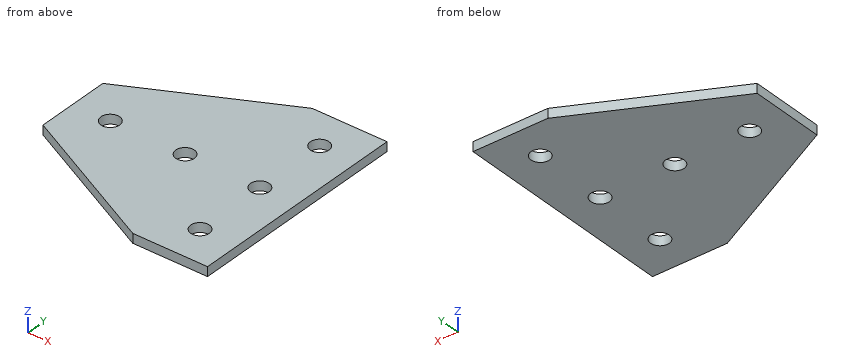
Autodesk Inventor part; units mm, degrees
ref_plane "YZ Plane" through (0, 0, 0) normal (1, 0, 0) x (0, 1, 0)
ref_plane "XZ Plane" through (0, 0, 0) normal (0, 1, 0) x (-1, 0, 0)
ref_plane "XY Plane" through (0, 0, 0) normal (0, 0, 1) x (1, 0, 0)
sketch "Sketch1" plane through (0, 0, 0) normal (0, 0, 1) x (1, 0, 0)
  line L0 (0, 0) -> (0, -76.2)
  line L1 (0, 0) -> (76.2, 0) construction
  line L2 (0, 0) -> (-25.4, 0)
  line L3 (-25.4, 0) -> (-76.2, -25.4)
  line L4 (-76.2, -25.4) -> (-76.2, -50.8)
  line L5 (-76.2, -50.8) -> (-25.4, -76.2)
  line L6 (-25.4, -76.2) -> (0, -76.2)
  circle A0 centre (-12.7, -12.7) radius 3.175
  circle A1 centre (-12.7, -38.1) radius 3.175
  circle A2 centre (-12.7, -63.5) radius 3.175
  circle A3 centre (-38.1, -38.1) radius 3.175
  circle A4 centre (-63.5, -38.1) radius 3.175
  dimension "d0" = 76.2
  dimension "d2" = 25.4
  dimension "d3" = 25.4
  dimension "d4" = 25.4
  dimension "d5" = 76.2
  dimension "d6" = 6.35
  dimension "d7" = 12.7
  dimension "d8" = 12.7
  dimension "d9" = 12.7
  dimension "d10" = 38.1
  dimension "d11" = 25.4
  dimension "d12" = 25.4
  dimension "d13" = 12.7
  dimension "d14" = 12.7
  dimension "d15" = 12.7
  dimension "d16" = 12.7
extrude "Extrusion1" add sketch "Sketch1" along normal blind 3.175
properties part number "15102898-16-P-0210" material "Aluminum 6061"
Work out the finished part from the listing and answer in its coordinate system (mm). Coordinates: 2 decimals unless noted, no trailing zeros. Loops run counter-clockwise (first coordinate to the right, second up) from the corner with the lowest first, then second, coordinate; pieces in that order, holes last. Notation, with made-up numbers: M 2,61.25 L 21,61.25 A7 ccw 21,66.25 Z; hole C 62.25,-4 d7. An arc over 180 degrees is marked long. Answer in a Markdown table with one row per item. Add a question column.
1. Find section C-C, the plane z = 2. Write down the section's boundary in (x, y) (3 decimals).
2. Find section B-B, the plane y = -12.7. Write down the section's boundary in (x, z) (3 decimals).
3. Find section A-A, the plane x = -39. Write down the section's boundary in (y, z) (3 decimals).
4. Find section D-D, the plane y = -38.1. Write down the section's boundary in (x, z) (3 decimals).
5. Consider L1, parallel to Y at x = -12.7, z = 0.75 (3 decimals); L2, parallel to X at y = -38, z = 0.7; L3, parallel to X at y = -68.5, z = 1.55. Determine where each line is inside the solid, lowest interval first.
6. A flat-ended cylindrical pin translates along its axis: P1, Ø4, axis at x = -12.7, y = -12.7, coming from the +Z side. Find the tip coordinate at first contact, or state that the pin passes through.
Reported:
| question | item | result |
|---|---|---|
| 1 | outline | M -76.2,-50.8 L -25.4,-76.2 L 0,-76.2 L 0,0 L -25.4,0 L -76.2,-25.4 Z; hole C -63.5,-38.1 d6.35; hole C -38.1,-38.1 d6.35; hole C -12.7,-63.5 d6.35; hole C -12.7,-38.1 d6.35; hole C -12.7,-12.7 d6.35 |
| 2 | outline | M -50.8,0 L -15.875,0 L -15.875,3.175 L -50.8,3.175 Z; M -9.525,0 L 0,0 L 0,3.175 L -9.525,3.175 Z |
| 3 | outline | M -69.4,0 L -41.145,0 L -41.145,3.175 L -69.4,3.175 Z; M -35.055,0 L -6.8,0 L -6.8,3.175 L -35.055,3.175 Z |
| 4 | outline | M -76.2,0 L -66.675,0 L -66.675,3.175 L -76.2,3.175 Z; M -60.325,0 L -41.275,0 L -41.275,3.175 L -60.325,3.175 Z; M -34.925,0 L -15.875,0 L -15.875,3.175 L -34.925,3.175 Z; M -9.525,0 L 0,0 L 0,3.175 L -9.525,3.175 Z |
| 5 | L1 | y = -76.2 to -66.675, -60.325 to -41.275, -34.925 to -15.875, -9.525 to 0 |
| 5 | L2 | x = -76.2 to -66.67, -60.33 to -41.27, -34.93 to -15.87, -9.53 to 0 |
| 5 | L3 | x = -40.8 to 0 |
| 6 | P1 | passes through |
